Autodesk Fusion 360 part; units mm, degrees
sketch "Sketch1" plane through (0, 0, 0) normal (0, 0, 1) x (1, 0, 0)
  line L0 (0, 0) -> (140, 0)
  line L1 (140, 0) -> (140, 210)
  line L2 (140, 210) -> (0, 210)
  line L3 (0, 210) -> (0, 0)
  dimension "d1" = 140
  dimension "d2" = 210
extrude "Extrude1" add sketch "Sketch1" along normal blind 6.35
sketch "Sketch2" plane through (0, 0, 6.35) normal (0, 0, 1) x (-1, 0, 0)
  line L0 (0, -210) -> (0, 0)
  line L1 (0, 0) -> (-140, 0)
  line L2 (-140, 0) -> (-140, -210)
  line L3 (-140, -210) -> (0, -210)
  circle A0 centre (-132.5, -7.5) radius 3.2
  line L4 (-140, -105) -> (0, -105)
  line L5 (-70, 0) -> (-70, -210)
  circle A1 centre (-7.5, -7.5) radius 3.2
  circle A2 centre (-132.5, -202.5) radius 3.2
  circle A3 centre (-7.5, -202.5) radius 3.2
  dimension "d5" = 6.4
  dimension "d6" = 7.5
  dimension "d7" = 7.5
extrude "Extrude2" cut sketch "Sketch2" against normal blind 10 contours A0 | A1 | A2 | A3
sketch "Sketch3" plane through (0, 0, 6.35) normal (0, 0, 1) x (-1, 0, 0)
  circle A0 centre (-7.5, -7.5) radius 3.2
  circle A1 centre (-7.5, -202.5) radius 3.2
  circle A2 centre (-132.5, -7.5) radius 3.2
  circle A3 centre (-132.5, -202.5) radius 3.2
  line L0 (0, -210) -> (0, 0)
  line L1 (0, 0) -> (-140, 0)
  line L2 (-140, 0) -> (-140, -210)
  line L3 (-140, -210) -> (0, -210)
  line L4 (0, -105) -> (-140, -105)
  circle A4 centre (-15, -105) radius 3
  circle A5 centre (-125, -105) radius 3
  dimension "d10" = 6
  dimension "d11" = 6
  dimension "d12" = 110
  dimension "d13" = 15
extrude "Extrude3" cut sketch "Sketch3" against normal blind 10 contours L4 A4 | L4 A4 | L4 A5 | L4 A5
Could you check a few things on this model? Use its own coordinates, in mm. Round coordinates to 2 decimals unless told otherwise and drop trailing zeros. Write each loop counter-clockwise with the first axis right and the second up, starting at its lowest first coordinate (ties: lowest second). Pieces come first, ordered by that corner, then holes. Notation, with made-up numbers: (89.5, 29.5) -> (116.5, 29.5) arc R23 cw to (116.5, 59.5) -> close; hole circle Ø6 at (20, 34.25). An arc over 180 degrees is marked (long way). Use a Markdown table: item, result.
1. If we section it at A-A (y = 105): List the corners of the cut face in (x, z) for me, then the cut area to 3 significant figures.
Answer key:
| item | result |
|---|---|
| outline | (0, 0) -> (12, 0) -> (12, 6.35) -> (0, 6.35) -> close; (18, 0) -> (122, 0) -> (122, 6.35) -> (18, 6.35) -> close; (128, 0) -> (140, 0) -> (140, 6.35) -> (128, 6.35) -> close |
| area | 813 mm^2 |
2. Please list where these lines run through material, in increasing order: probe 1 along Y at (x, z) = (7.5, 4.5); probe 2 along X at (y, z) = (105, 1.5); probe 3 along X at (y, z) = (202.5, 2.5).
Answer key:
| item | result |
|---|---|
| probe 1 | y = 0 to 4.3, 10.7 to 199.3, 205.7 to 210 |
| probe 2 | x = 0 to 12, 18 to 122, 128 to 140 |
| probe 3 | x = 0 to 4.3, 10.7 to 129.3, 135.7 to 140 |
3. We'd pull the mould along Y, two halves only. Please class faces 1 (the face through (71, 210, 3)), 2 (the face through (7.917, 199.327, 3.219)), 3 (the face through (69, 106, 6.35)): +Y half, -Y half, draft (parallel to the pull), parting line (faces both ways), or undercut.
Answer key:
| item | result |
|---|---|
| face 1 | +Y half |
| face 2 | undercut |
| face 3 | draft |
4. For pin 1 Ø4 at (x, y) = (132.5, 202.5) entering from +Z, with a flat end and sliding along its axis, tell me the tip position at first contact or that it passes through.
Answer key:
| item | result |
|---|---|
| pin 1 | passes through |
5. If we section it at B-B (x = 125): List the corners of the cut face in (y, z) for me.
Answer key:
| item | result |
|---|---|
| outline | (0, 0) -> (102, 0) -> (102, 6.35) -> (0, 6.35) -> close; (108, 0) -> (210, 0) -> (210, 6.35) -> (108, 6.35) -> close |
6. If we section it at C-C (x = 7.5): List the corners of the cut face in (y, z) for me.
Answer key:
| item | result |
|---|---|
| outline | (0, 0) -> (4.3, 0) -> (4.3, 6.35) -> (0, 6.35) -> close; (10.7, 0) -> (199.3, 0) -> (199.3, 6.35) -> (10.7, 6.35) -> close; (205.7, 0) -> (210, 0) -> (210, 6.35) -> (205.7, 6.35) -> close |
